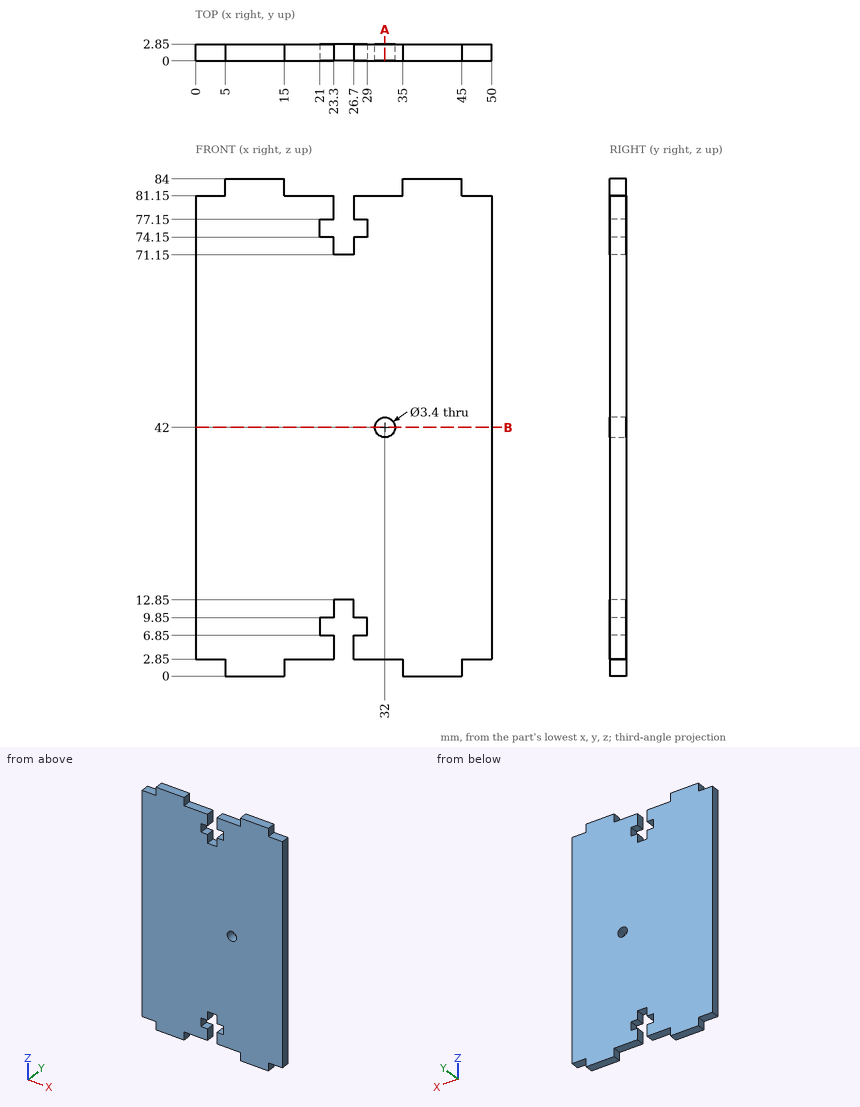
Geometry: see drawing. Coordinates: mm, zero at the bounding-box minimum. Round coordinates to 2 decimals unless told otherwise and drop trailing zeros. Loops run counter-clockwise (first coordinate to the right, second up) from the corner with the lowest first, then second, coordinate; pieces in that order, holes last. Notation, with made-up numbers: (82.5, 87.5) -> (123.5, 87.5) arc R25 ccw to (123.5, 118.5) -> close; hole circle Ø10 at (76, 72.25). An arc over 180 degrees is marked (long way). Use one line per item in the form item = value. Start each with the question number.
Item 1: Contact query for flat-ended pins moving along their axis: pin 1 Ø1.4 at (y, z) = (1, 82.5) entering from -X; pin 2 Ø0.9 at (x, y) = (47, 0.5) entering from -Z; pin 3 Ø1.2 at (x, y) = (22, 1.5) entering from +Z. Output: stop coordinate, or through.
Item 2: Material intervals for L1, parallel to X at y = 0.35, z = 8; L2, parallel to X at y = 1.9, z = 42; L3, parallel to Z at x = 31, y = 2.2, sorted ascending. Write a range as from..to.
Item 3: Section query A-A on x = 32. Return the cut outline in (y, z).
Item 4: Section query B-B on z = 42. Return the cut outline in (x, y).
Ans:
q1.pin_1 = 5
q1.pin_2 = 2.85
q1.pin_3 = 81.15
q2.L1 = 0..21, 29..50
q2.L2 = 0..30.3, 33.7..50
q2.L3 = 2.85..40.63, 43.37..81.15
q3.outline = (0, 2.85) -> (2.85, 2.85) -> (2.85, 40.3) -> (0, 40.3) -> close; (0, 43.7) -> (2.85, 43.7) -> (2.85, 81.15) -> (0, 81.15) -> close
q4.outline = (0, 0) -> (30.3, 0) -> (30.3, 2.85) -> (0, 2.85) -> close; (33.7, 0) -> (50, 0) -> (50, 2.85) -> (33.7, 2.85) -> close
